Build history of the part. All positions in model axes, mm. A direction names the side the tool comes from. Round coordinates to 2 decimals unless told otherwise and drop trailing zeros. Write each loop counter-clockwise with the first axis right and the second up, starting at its lowest first coordinate (ties: lowest second). Pieces come first, ordered by that corner, then holes. Notation, with made-up numbers: (67, 6) -> (93, 6) arc R15 cw to (93, 15) -> close; hole circle Ø7 at (29, 35.5). An arc over 180 degrees is marked (long way). Answer in a Markdown table with one row per item. Add a question column.
from build123d import *

# Parameters (mm, degrees)
F0_W     = 33.02
F0_H     = 2.159
F0_R     = 2.54
F1_DEPTH = 3.683
F2_DEPTH = 13.335
F3_DEPTH = 6.985
F4_R     = 1.778
F5_DEPTH = 25.4
F6_R     = 2.54
F8_R     = 1.0795
F9_DEPTH = 3.81


with BuildPart() as f1:
    # F0 (on Top) → F1 (new body)
    with BuildSketch(Plane.XY):
        with Locations((12.518704, 1.0795)):
            Rectangle(F0_W, F0_H)
        with BuildLine():
            Line((7.949625, 26.731342), (-3.991296, 2.159))
            Line((-3.991296, 2.159), (29.028704, 2.159))
            Line((29.028704, 2.159), (17.087783, 26.731342))
            ThreePointArc((17.087783, 26.731342), (17.469326, 25.650184), (17.598704, 24.511))
            ThreePointArc((17.598704, 24.511), (11.37952, 19.560378), (7.949625, 26.731342))
        make_face()
        with BuildLine():
            ThreePointArc((17.087783, 26.731342), (12.518704, 29.591), (7.949625, 26.731342))
            ThreePointArc((7.949625, 26.731342), (11.37952, 19.560378), (17.598704, 24.511))
            ThreePointArc((17.598704, 24.511), (17.469326, 25.650184), (17.087783, 26.731342))
        make_face()
        with Locations((12.518704, 24.511)):
            Circle(F0_R, mode=Mode.SUBTRACT)
    extrude(amount=F1_DEPTH)

    # F0 (on Top) → F2 (join)
    with BuildSketch(Plane.XY):
        with Locations((12.518704, 1.0795)):
            Rectangle(F0_W, F0_H)
    extrude(amount=F2_DEPTH)

    # F0 (on Top) → F3 (join)
    with BuildSketch(Plane.XY):
        with BuildLine():
            ThreePointArc((17.087783, 26.731342), (12.518704, 29.591), (7.949625, 26.731342))
            ThreePointArc((7.949625, 26.731342), (11.37952, 19.560378), (17.598704, 24.511))
            ThreePointArc((17.598704, 24.511), (17.469326, 25.650184), (17.087783, 26.731342))
        make_face()
        with Locations((12.518704, 24.511)):
            Circle(F0_R, mode=Mode.SUBTRACT)
    extrude(amount=F3_DEPTH)

    # F4 (on face) → F5 (cut)
    with BuildSketch(Plane(origin=(0, 2.159, 0), x_dir=(-1, 0, 0), z_dir=(0, 1, 0))):
        with Locations((0.816296, 9.730688)):
            Circle(F4_R)
        with Locations((-25.853704, 9.730688)):
            Circle(F4_R)
        with Locations((-17.979704, 9.730688)):
            Circle(F4_R)
        with Locations((-7.057704, 9.730688)):
            Circle(F4_R)
    extrude(amount=-F5_DEPTH, mode=Mode.SUBTRACT)

    # F6
    f6_edges = [f1.edges().sort_by_distance(p)[0] for p in [
        (-3.991296, 1.0795, 13.335),
        (29.028704, 1.0795, 13.335),
    ]]
    fillet(f6_edges, radius=F6_R)

    # F8 (on offset) → F9 (cut)
    with BuildSketch(Plane.XZ.offset(-29.591)):
        with Locations((12.518704, 3.4925)):
            Circle(F8_R)
    extrude(amount=F9_DEPTH, mode=Mode.SUBTRACT)


solid = f1.part
(1) Saw through at B-B (y = 23). List the corners of the cut face in (x, z) (3 decimals).
(2) Saw through at A-A (z = 5.5). List the corners of the cut face in (x, y).
(3) Which spindle directions (+Z, -Z, +X, -X, +Y, -Y) get a long thin tool onto all of the face, cutting with end or side? Do faces 5 (the face through (12.378, 28.22, 4.563)), 6 (the face through (14, 27, 6.985)), 7 (the face through (11.97, 22.03, 3.44)), 8 (the face through (12, 1, 13.335)), 9 (the face through (12, 2.159, 8)). Say none if no direction does.
(4) Mould opens along Z. For faces 1 (the face through (-3.991, 1, 5)), 2 (the face through (7.289, 1.095, 11.494)), 3 (the face through (28.304, 1.095, 12.571)), 4 (the face through (26.085, 1.095, 11.494)) say: pulls with the +Z half, pulls with the -Z half, needs draft (parallel to the pull), parting line crosses it, or undercut.
(5) Saw through at D-D (y = 4.5). List the corners of the cut face in (x, z).
(6) Drop flat-ended pins along their axis: P1, Ø3, axis at x = 14, y = 24, coming from the +Z side (3 decimals); P2, Ø8, axis at x = 6, z = 7.5, coming from the +Y side; P3, Ø1, axis at x = 1, z = 6, coming from the -Y side; P4, Ø6, axis at y = 20, z = 6.5, coming from the -X side. Give the stop position or say it passes through.
(7) Probe line 1 along Z through (x, y) = (14, 16.75); line 2 along Y through (x, z) = (1, 7); line 3 along Y through (x, z) = (13.5, 1.5). List the from-to ranges inside material, lowest first.
(8) Saw through at C-C (x = 14). List the corners of the cut face in (y, z) (3 decimals).
Answer sheet:
| question | item | result |
|---|---|---|
| 1 | outline | (6.136, 0) -> (10.477, 0) -> (10.477, 6.985) -> (7.669, 6.985) -> (7.669, 3.683) -> (6.136, 3.683) -> close; (14.56, 0) -> (18.901, 0) -> (18.901, 3.683) -> (17.369, 3.683) -> (17.369, 6.985) -> (14.56, 6.985) -> close |
| 2 | outline | (-3.99, 0) -> (29.03, 0) -> (29.03, 2.16) -> (-3.99, 2.16) -> close; (17.09, 26.73) arc R5.08 ccw (long way) to (17.6, 24.51) arc R5.08 ccw to start; hole circle Ø5.08 at (12.52, 24.51) |
| 3 | face 5 | +Y |
| 3 | face 6 | +Z, +X, -X, +Y |
| 3 | face 7 | +Z, -Z |
| 3 | face 8 | +Z, +X, -X, +Y, -Y |
| 3 | face 9 | +Z, +X, -X |
| 4 | face 1 | needs draft |
| 4 | face 2 | undercut |
| 4 | face 3 | pulls with the +Z half |
| 4 | face 4 | undercut |
| 5 | outline | (-2.85, 0) -> (27.89, 0) -> (27.89, 3.68) -> (-2.85, 3.68) -> close |
| 6 | P1 | stops at z = 6.985 |
| 6 | P2 | stops at y = 28.9 |
| 6 | P3 | stops at y = 0 |
| 6 | P4 | stops at x = 4.18 |
| 7 | line 1 | z = 0 to 3.68 |
| 7 | line 2 | y = 0 to 2.16 |
| 7 | line 3 | y = 0 to 22.17, 26.85 to 29.5 |
| 8 | outline | (0, 0) -> (22.448, 0) -> (22.448, 6.985) -> (19.652, 6.985) -> (19.652, 3.683) -> (2.159, 3.683) -> (2.159, 13.335) -> (0, 13.335) -> close; (26.574, 0) -> (29.37, 0) -> (29.37, 6.985) -> (26.574, 6.985) -> close |
